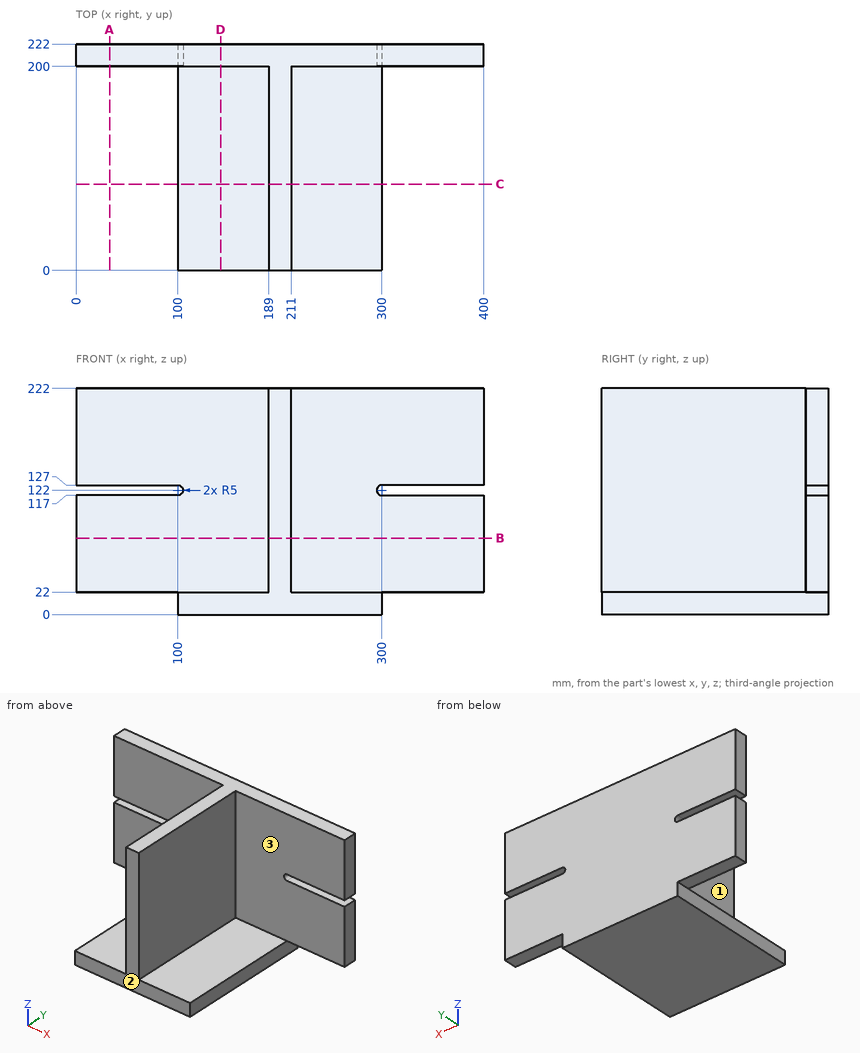
Input: dimensioned drawing with shaded views. Units: mm. Origin: part minimum x, y, z. A direction names the side the tool comes from. Round coordinates to 2 decimals unless told otherwise and drop trailing zeros. Loops run counter-clockwise (first coordinate to the right, second up) from the corner with the lowest first, then second, coordinate; pieces in that order, holes last.
1) Section query D-D on x = 142. Return the cut outline in (y, z), plus the area to 3 significant figures.
Ans:
outline: (0, 0) - (222, 0) - (222, 222) - (200, 222) - (200, 22) - (0, 22) - close
area: 9,280 mm2
2) Section query A-A on x = 33. Return the cut outline in (y, z), plus the area to 3 significant figures.
Ans:
outline: (200, 22) - (222, 22) - (222, 117) - (200, 117) - close; (200, 127) - (222, 127) - (222, 222) - (200, 222) - close
area: 4,180 mm2
3) Material intervals for line 1 (X direction, y = 158, z = 206); line 2 (Z direction, x = 181.5, y = 171.5); line 3 (Y direction, x = 163, z = 71), sorted ascending.
Ans:
line 1: x = 189 to 211
line 2: z = 0 to 22
line 3: y = 200 to 222
4) Pin query (flat end, axial travel): pin 1 (8 mm diameter, centred on x = 247.5, y = 189.5, fed in from -Z); pin 2 (24 mm diameter, centred on x = 39, y = 216, fed in from -Z); pin 3 (1 mm diameter, centred on y = 22, z = 121.5, fed in from -X); pin 4 (11 mm diameter, centred on y = 83, z = 13.5, fed in from +X). Return the tip coordinate at first contact, or that it passes through.
Ans:
pin 1: stops at z = 0
pin 2: stops at z = 22
pin 3: stops at x = 189
pin 4: stops at x = 300
5) Section query B-B on z = 75. Return the cut outline in (x, y), plus the area to 3 significant figures.
Ans:
outline: (0, 200) - (189, 200) - (189, 0) - (211, 0) - (211, 200) - (400, 200) - (400, 222) - (0, 222) - close
area: 13,200 mm2
6) Section query C-C on y = 84.5. Return the cut outline in (x, z), plus the area to 3 significant figures.
Ans:
outline: (100, 0) - (300, 0) - (300, 22) - (211, 22) - (211, 222) - (189, 222) - (189, 22) - (100, 22) - close
area: 8,800 mm2
7) Set-up query: the marked faces 1, 2 and 3. Return all of +Z, -Z, +X, -X, +Y, -Y with unobstructed straight access to the full face (end or side cutting, diameter ignored); none if empty.
Ans:
face 1: +Z, -X, -Y
face 2: +Z, -Z, +X, -X, -Y
face 3: +Z, +X, -Y
